```python
from build123d import *

# Parameters (mm, degrees)
CUT_EXTRUDE1_DEPTH = 3.81
FILLET1_R          = 0.762
SCALE1_SCALE       = 3


with BuildPart() as part:
    # Sketch1 → Revolve1 (revolve)
    with BuildSketch(Plane.XY, mode=Mode.PRIVATE) as revolve1_sk:
        with BuildLine():
            Line((0, 0), (57.15, 0))
            Line((57.15, 0), (57.15, 3.81))
            Line((57.15, 3.81), (8.89, 3.81))
            Line((8.89, 3.81), (8.89, 8.255))
            ThreePointArc((8.89, 8.255), (2.818084231, 5.879563136), (0, 0))
        make_face()
    revolve(revolve1_sk.sketch.rotate(Axis((0, 0, 0), (1, 0, 0)), 90), axis=Axis((0, 0, 0), (1, 0, 0)))

    # Sketch3 → Cut-Extrude1 (cut)
    with BuildSketch(Plane(origin=(0, 0, 0), x_dir=(0, 0, -1), z_dir=(1, 0, 0))):
        with BuildLine():
            Line((1.905, -3.661588624), (1.905, -6.985))
            Line((1.905, -6.985), (-1.905, -6.985))
            Line((-1.905, -6.985), (-1.905, -3.661588624))
            ThreePointArc((-1.905, -3.661588624), (-3.829921876, 0), (-1.905, 3.661588624))
            Line((-1.905, 3.661588624), (-1.905, 6.985))
            Line((-1.905, 6.985), (1.905, 6.985))
            Line((1.905, 6.985), (1.905, 3.661588624))
            ThreePointArc((1.905, 3.661588624), (3.829921876, 0), (1.905, -3.661588624))
        make_face()
    extrude(amount=CUT_EXTRUDE1_DEPTH, mode=Mode.SUBTRACT)

    # Fillet1
    fillet1_edges = [part.edges().sort_by_distance(p)[0] for p in [
        (8.89, 0, -8.255),
        (57.15, 0, -3.81),
    ]]
    fillet(fillet1_edges, radius=FILLET1_R)


with BuildPart() as part_1:
    # Scale1: scaled about (24.334751601, 6e-09, -5e-09)
    add(part.part.scale(SCALE1_SCALE).moved(Location((-48.669503202, -1.2e-08, 1e-08))))


solid = part_1.part
```
For this review, take the finished solid that the model builds, in its own axes (mm). A direction names the side the tool comes from. Give positions to 0.01 mm unless a question says otherwise; leave off trailing zeros. Order: outer loops, then holes, each group sorted by start corner. A loop starts at its lowest first (then second) coordinate and runs counter-clockwise, first axis right, second up.
1) The part is to be moulded in two halves that separate along Z. For faces 4 (the face through (-22, 5.4, 10.3)), 5 (the face through (-40, -14, 5.715)), 6 (the face through (48.25, 10.14, 5.274)), say which applies: released by +Z, released by -Z, zero draft, split by the parting line, or undercut.
2) Insertion check: pin 1 (5 mm diameter, centred on x = 82, z = 14, fed in from -Y); pin 2 (12 mm diameter, centred on x = 103, y = 3.5, fed in from -Z); pin 3 (8 mm diameter, centred on x = -41.5, y = -16, fed in from -Z); pin 4 (8 mm diameter, centred on x = -41.5, y = -15, fed in from +Z). Each pin has a flat end and moves straight along its axis. Give the tip position at first contact, or say it passes through.
3) Wall thickness on line 1 (X direction, y = 4.5, z = -6); line 2 (X direction, y = -17, z = 2); line 3 (Y direction, x = 48.5, z = -1.5): over which ranges is each line inside the solid? List them lowest first.
4) For faces 1 (the face through (-40, -14, -5.715)), 2 (the face through (-37.24, 0, 0)), 3 (the face through (122.78, 0, 0)), list the 3-axis set-ups (+Z, -Z, +X, -X, +Y, -Y) from which the entire face can be reached by the end or side of a thin tool; tool diameter is ignored.
5) Take a section at A-A (x = 55.5). Give the boundary of the cut face in (y, z), then the cut area to 3 significant figures.
Derived:
1. face 4: zero draft
1. face 5: undercut
1. face 6: split by the parting line
2. pin 1: passes through
2. pin 2: stops at z = -11.43
2. pin 3: stops at z = -13.66
2. pin 4: stops at z = 14.57
3. line 1: x = -37.24 to 122.78
3. line 2: x = -37.24 to -22
3. line 3: y = -11.33 to 11.33
4. face 1: -X, +Y, -Y
4. face 2: -X
4. face 3: +Z, -Z, +X, +Y, -Y
5. outline: circle Ø22.86 at (0, 0)
5. area: 410 mm2
